Design review of the part built by this model. Coordinates are the model's own, in mm. Face numbers are marked on the shaded views. A direction names the side the tool comes from. Give positions to 0.01 mm unless a question says otherwise; leave off trailing zeros. Order: outer loops, then holes, each group sorted by start corner. A loop starts at its lowest first (then second) coordinate and runs counter-clockwise, first axis right, second up.
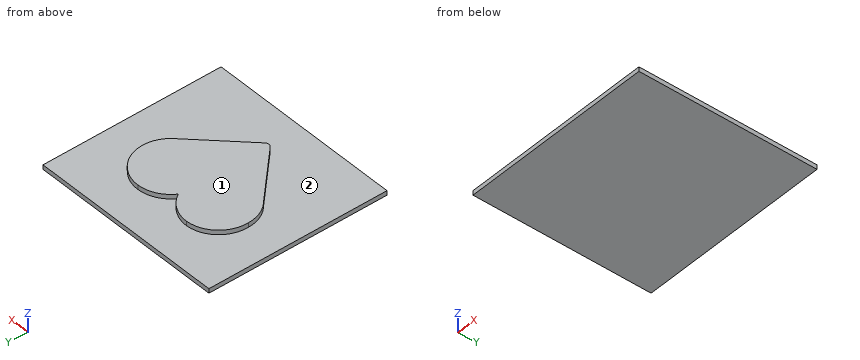
```python
from build123d import *

# Parameters (mm, degrees)
F0_W      = 137.7741502185
F0_H      = 127
F1_DEPTH  = 6.35
F1_FACE_W = 137.7741502185
F1_FACE_H = 127
F2_DEPTH  = 3.175


# Not quite as in the source:
# - a length typed as a fraction of an inch, garbled in the dataset ("3 / 203.2 mm" for 3/8 in), is restored


with BuildPart() as f1:
    # F0 (on Top) → F1 (new body)
    with BuildSketch(Plane.XY):
        Rectangle(F0_W, F0_H)
        with BuildLine():
            add(Edge.make_bspline(
                [(43.4870751092, 14.3433300558), (43.4870751092, 27.462876741), (32.8514196183, 38.0979859262), (19.7318729331, 38.0979859262)],
                knots=[0, 0, 0, 0, 1, 1, 1, 1], degree=3))
            add(Edge.make_bspline(
                [(35.3328363694, -3.5415767003), (40.3215229837, 0.8101175052), (43.4870751092, 7.2004637855), (43.4870751092, 14.3433300558)],
                knots=[0, 0, 0, 0, 1, 1, 1, 1], degree=3))
            Line((35.3328363694, -3.5415767003), (1.7854201908, -37.2041767762))
            add(Edge.make_bspline(
                [(-0.3831377338, -38.1), (0.4300700378, -38.1007554216), (1.2100121742, -37.7785167454), (1.7854201908, -37.2041767762)],
                knots=[0, 0, 0, 0, 1, 1, 1, 1], degree=3))
            add(Edge.make_bspline(
                [(-2.5508625567, -37.2021627024), (-1.9759883158, -37.7770369433), (-1.1963458563, -38.1), (-0.3831377338, -38.1)],
                knots=[0, 0, 0, 0, 1, 1, 1, 1], degree=3))
            Line((-2.5508625567, -37.2021627024), (-35.3333666072, -4.280217526))
            add(Edge.make_bspline(
                [(-43.4870751092, 13.6046892301), (-43.4870751092, 6.4618229599), (-40.3218925434, 0.0714766795), (-35.3333666072, -4.280217526)],
                knots=[0, 0, 0, 0, 1, 1, 1, 1], degree=3))
            add(Edge.make_bspline(
                [(-20.4995127814, 38.1), (-33.6124722867, 37.6843099249), (-43.9027651844, 26.7176487354), (-43.4870751092, 13.6046892301)],
                knots=[0, 0, 0, 0, 1, 1, 1, 1], degree=3))
            add(Edge.make_bspline(
                [(-0.3831377338, 26.5499493108), (-4.4942474015, 33.3906018689), (-11.9332866772, 38.0146472183), (-20.4995127814, 38.1)],
                knots=[0, 0, 0, 0, 1, 1, 1, 1], degree=3))
            add(Edge.make_bspline(
                [(19.7318729331, 38.0979859262), (11.16547776, 38.0134786667), (3.7291785921, 33.3902005219), (-0.3831377338, 26.5499493108)],
                knots=[0, 0, 0, 0, 1, 1, 1, 1], degree=3))
        make_face(mode=Mode.SUBTRACT)
        with BuildLine():
            add(Edge.make_bspline(
                [(35.3328363694, -3.5415767003), (40.3215229837, 0.8101175052), (43.4870751092, 7.2004637855), (43.4870751092, 14.3433300558)],
                knots=[0, 0, 0, 0, 1, 1, 1, 1], degree=3))
            add(Edge.make_bspline(
                [(43.4870751092, 14.3433300558), (43.4870751092, 27.462876741), (32.8514196183, 38.0979859262), (19.7318729331, 38.0979859262)],
                knots=[0, 0, 0, 0, 1, 1, 1, 1], degree=3))
            add(Edge.make_bspline(
                [(19.7318729331, 38.0979859262), (11.16547776, 38.0134786667), (3.7291785921, 33.3902005219), (-0.3831377338, 26.5499493108)],
                knots=[0, 0, 0, 0, 1, 1, 1, 1], degree=3))
            add(Edge.make_bspline(
                [(-0.3831377338, 26.5499493108), (-4.4942474015, 33.3906018689), (-11.9332866772, 38.0146472183), (-20.4995127814, 38.1)],
                knots=[0, 0, 0, 0, 1, 1, 1, 1], degree=3))
            add(Edge.make_bspline(
                [(-20.4995127814, 38.1), (-33.6124722867, 37.6843099249), (-43.9027651844, 26.7176487354), (-43.4870751092, 13.6046892301)],
                knots=[0, 0, 0, 0, 1, 1, 1, 1], degree=3))
            add(Edge.make_bspline(
                [(-43.4870751092, 13.6046892301), (-43.4870751092, 6.4618229599), (-40.3218925434, 0.0714766795), (-35.3333666072, -4.280217526)],
                knots=[0, 0, 0, 0, 1, 1, 1, 1], degree=3))
            Line((-35.3333666072, -4.280217526), (-2.5508625567, -37.2021627024))
            add(Edge.make_bspline(
                [(-2.5508625567, -37.2021627024), (-1.9759883158, -37.7770369433), (-1.1963458563, -38.1), (-0.3831377338, -38.1)],
                knots=[0, 0, 0, 0, 1, 1, 1, 1], degree=3))
            add(Edge.make_bspline(
                [(-0.3831377338, -38.1), (0.4300700378, -38.1007554216), (1.2100121742, -37.7785167454), (1.7854201908, -37.2041767762)],
                knots=[0, 0, 0, 0, 1, 1, 1, 1], degree=3))
            Line((1.7854201908, -37.2041767762), (35.3328363694, -3.5415767003))
        make_face()
    extrude(amount=-F1_DEPTH)

    # F0 (on Top) + F1_face (on face) → F2 (cut)
    with BuildSketch(Plane.XY):
        Rectangle(F0_W, F0_H)
        with BuildLine():
            add(Edge.make_bspline(
                [(43.4870751092, 14.3433300558), (43.4870751092, 27.462876741), (32.8514196183, 38.0979859262), (19.7318729331, 38.0979859262)],
                knots=[0, 0, 0, 0, 1, 1, 1, 1], degree=3))
            add(Edge.make_bspline(
                [(35.3328363694, -3.5415767003), (40.3215229837, 0.8101175052), (43.4870751092, 7.2004637855), (43.4870751092, 14.3433300558)],
                knots=[0, 0, 0, 0, 1, 1, 1, 1], degree=3))
            Line((35.3328363694, -3.5415767003), (1.7854201908, -37.2041767762))
            add(Edge.make_bspline(
                [(-0.3831377338, -38.1), (0.4300700378, -38.1007554216), (1.2100121742, -37.7785167454), (1.7854201908, -37.2041767762)],
                knots=[0, 0, 0, 0, 1, 1, 1, 1], degree=3))
            add(Edge.make_bspline(
                [(-2.5508625567, -37.2021627024), (-1.9759883158, -37.7770369433), (-1.1963458563, -38.1), (-0.3831377338, -38.1)],
                knots=[0, 0, 0, 0, 1, 1, 1, 1], degree=3))
            Line((-2.5508625567, -37.2021627024), (-35.3333666072, -4.280217526))
            add(Edge.make_bspline(
                [(-43.4870751092, 13.6046892301), (-43.4870751092, 6.4618229599), (-40.3218925434, 0.0714766795), (-35.3333666072, -4.280217526)],
                knots=[0, 0, 0, 0, 1, 1, 1, 1], degree=3))
            add(Edge.make_bspline(
                [(-20.4995127814, 38.1), (-33.6124722867, 37.6843099249), (-43.9027651844, 26.7176487354), (-43.4870751092, 13.6046892301)],
                knots=[0, 0, 0, 0, 1, 1, 1, 1], degree=3))
            add(Edge.make_bspline(
                [(-0.3831377338, 26.5499493108), (-4.4942474015, 33.3906018689), (-11.9332866772, 38.0146472183), (-20.4995127814, 38.1)],
                knots=[0, 0, 0, 0, 1, 1, 1, 1], degree=3))
            add(Edge.make_bspline(
                [(19.7318729331, 38.0979859262), (11.16547776, 38.0134786667), (3.7291785921, 33.3902005219), (-0.3831377338, 26.5499493108)],
                knots=[0, 0, 0, 0, 1, 1, 1, 1], degree=3))
        make_face(mode=Mode.SUBTRACT)
    with BuildSketch(Plane(origin=(0, 0, -6.35), x_dir=(1, 0, 0), z_dir=(0, 0, -1))):
        Rectangle(F1_FACE_W, F1_FACE_H)
    extrude(amount=-F2_DEPTH, dir=(0, 0, 1), mode=Mode.SUBTRACT)


solid = f1.part
```
1. Take a section at B-B (y = -55). State the section outline as (x, z) points (3 decimals).
Recorded:
outline: (-68.887, -6.35) - (68.887, -6.35) - (68.887, -3.175) - (-68.887, -3.175) - close
2. For line 1 along Z through (x, y) = (61, -28) (3 decimals); line 2 along X through (y, z) = (30, -1.25); line 3 along Y through (x, z) = (15.5, -0.5), list the stretches that pass through material, from the lowest coordinate up.
Recorded:
line 1: z = -6.35 to -3.175
line 2: x = -37.62 to -2.9, 2.13 to 37.6
line 3: y = -23.44 to 37.68
3. Machinability: for the marked faces 1 and 2, which of the approach directions +Z, -Z, +X, -X, +Y, -Y give a long, thin tool a straight path to every point of the face, cutting with its end or side? Answer none if there is none.
Recorded:
face 1: +Z, +X, -X, +Y, -Y
face 2: +Z
4. Take a section at A-A (y = -26.5). State the section outline as (x, z) points (3 decimals), then the cut area to 3 significant figures.
Recorded:
outline: (-68.887, -6.35) - (68.887, -6.35) - (68.887, -3.175) - (12.453, -3.175) - (12.453, 0) - (-13.208, 0) - (-13.208, -3.175) - (-68.887, -3.175) - close
area: 519 mm2
